Could you check a few things on this model? Use its own coordinates, in mm. A direction names the side the tool comes from. Give positions to 0.01 mm unless a question says otherwise; leave off trailing zeros. Write each loop counter-clockwise with the first axis right and the second up, starting at its lowest first coordinate (ties: lowest second). Pieces come first, ordered by that corner, then holes. Notation, with made-up numbers: M 12,88.5 L 38,88.5 A18 ccw 38,100.5 Z; hole C 2,71 d3. An arc over 180 degrees is marked long. Answer as CSV lines item,"result". Start each with the question number.
from build123d import *

# Parameters (mm, degrees)
F0_R     = 280
F0_R_2   = 200
F1_DEPTH = 28
F4_R     = 13.5
F5_DEPTH = 28


with BuildPart() as f1:
    # F0 (on Top) → F1 (new body)
    with BuildSketch(Plane.XY):
        Circle(F0_R)
        Circle(F0_R_2, mode=Mode.SUBTRACT)
    extrude(amount=F1_DEPTH)

    # F2 (on Front) → F3 (revolve)
    with BuildSketch(Plane.XZ):
        with BuildLine():
            Line((200, -46.641016), (200, 28))
            Line((200, 28), (197, 28))
            Line((197, 28), (197, -46.641016))
            ThreePointArc((197, -46.641016), (196.420739, -51.04094), (194.722432, -55.141016))
            Line((194.722432, -55.141016), (18.267949, -360.769145))
            Line((18.267949, -360.769145), (0, -360.769145))
            Line((0, -360.769145), (0, -363.769145))
            Line((0, -363.769145), (20, -363.769145))
            Line((20, -363.769145), (197.320508, -56.641016))
            ThreePointArc((197.320508, -56.641016), (199.318517, -51.817397), (200, -46.641016))
        make_face()
    revolve(axis=Axis((0, 0, -362.269145), (0, 0, -1)))

    # F4 (on face) → F5 (cut, through all)
    with BuildSketch(Plane.XY.offset(28)):
        with Locations((255, 0)):
            Circle(F4_R)
        with Locations((235.589281, 97.584275)):
            Circle(F4_R)
        with Locations((180.312229, 180.312229)):
            Circle(F4_R)
        with Locations((97.584275, 235.589281)):
            Circle(F4_R)
        with Locations((0, 255)):
            Circle(F4_R)
        with Locations((-97.584275, 235.589281)):
            Circle(F4_R)
        with Locations((-180.312229, 180.312229)):
            Circle(F4_R)
        with Locations((-235.589281, 97.584275)):
            Circle(F4_R)
        with Locations((-255, 0)):
            Circle(F4_R)
        with Locations((-235.589281, -97.584275)):
            Circle(F4_R)
        with Locations((-180.312229, -180.312229)):
            Circle(F4_R)
        with Locations((-97.584275, -235.589281)):
            Circle(F4_R)
        with Locations((0, -255)):
            Circle(F4_R)
        with Locations((97.584275, -235.589281)):
            Circle(F4_R)
        with Locations((180.312229, -180.312229)):
            Circle(F4_R)
        with Locations((235.589281, -97.584275)):
            Circle(F4_R)
    extrude(amount=-F5_DEPTH, mode=Mode.SUBTRACT)


solid = f1.part
1. Please list where these lines run through material, in increasing order: line 1 (Y direction, x = 0, z = -31); line 2 (Z direction, x = 146.5, y = -238).
2. Thinking about a two-plate mould opening in X: for faces 1 (the cylindrical face through (190.764, -60.075, -22.994)), 2 (the cylindrical face through (-242.123, 4.055, 14.196)), 3 (the flat face through (-188, 84, 0)), which applies, pulls with the +X half, pulls with the -X half, needs draft (parallel to the pull), parting line crosses it, or undercut?
3. Imagine slicing it at C-C, the plane x = -230. Please give me the cut outline in (y, z), plus the area to 3 significant figures.
4. Imagine slicing it at D-D, the plane z = -116. Please give me the cut outline in (x, y), plus the area to 3 significant figures.
5. Will these pins go through, and if not, where does the flat tip stop? P1, Ø6, axis at x = -8, z = -167.5, coming from the +Y side; P2, Ø1, axis at x = -46.5, z = -77, coming from the +Y side; P3, Ø24.5, axis at x = -180.31, y = 180.31, coming from the -Z side; P4, Ø3, axis at x = 150, y = -14, coming from the -Z side.
6. Imagine slicing it at A-A, the plane y = 0. Please give me the cut outline in (x, z), plus the area to 3 significant figures.
7. On a 3-axis mill with a long thin cutter (end or side, diameter ignored), from which of +Z, -Z, +X, -X, +Y, -Y can I reach the whole of each face in a straight line? I mean faces 4 (the cylindrical face through (-246.3, -105.8, 14.2)), 5 (the cylindrical face through (187.903, -59.173, -9.843)). Say none if no direction works.
Solutions:
1,line 1,"-200 to -197, 197 to 200"
1,line 2,"0 to 28"
2,face 1,"parting line crosses it"
2,face 2,"undercut"
2,face 3,"needs draft"
3,outline,"M -159.69,0 L -109.87,0 L -109.87,28 L -159.69,28 Z; M -85.3,0 L 85.3,0 L 85.3,28 L -85.3,28 Z; M 109.87,0 L 159.69,0 L 159.69,28 L 109.87,28 Z"
3,area,"7,570 mm²"
4,outline,"C 0,0 d326.1; hole C 0,0 d319.17"
4,area,"3,510 mm²"
5,P1,"y = 134.82"
5,P2,"y = 179.97"
5,P3,"through"
5,P4,"z = -140.07"
6,outline,"M -280,0 L -268.5,0 L -268.5,28 L -280,28 Z; M -241.5,0 L -200,0 L -200,-46.64 A20 ccw -197.32,-56.64 L -20,-363.77 L 20,-363.77 L 197.32,-56.64 A20 ccw 200,-46.64 L 200,0 L 241.5,0 L 241.5,28 L 197,28 L 197,-46.64 A17 cw 194.72,-55.14 L 18.27,-360.77 L -18.27,-360.77 L -194.72,-55.14 A17 cw -197,-46.64 L -197,28 L -241.5,28 Z; M 268.5,0 L 280,0 L 280,28 L 268.5,28 Z"
6,area,"5,710 mm²"
7,face 4,"+Z, -Z"
7,face 5,"+Z"
